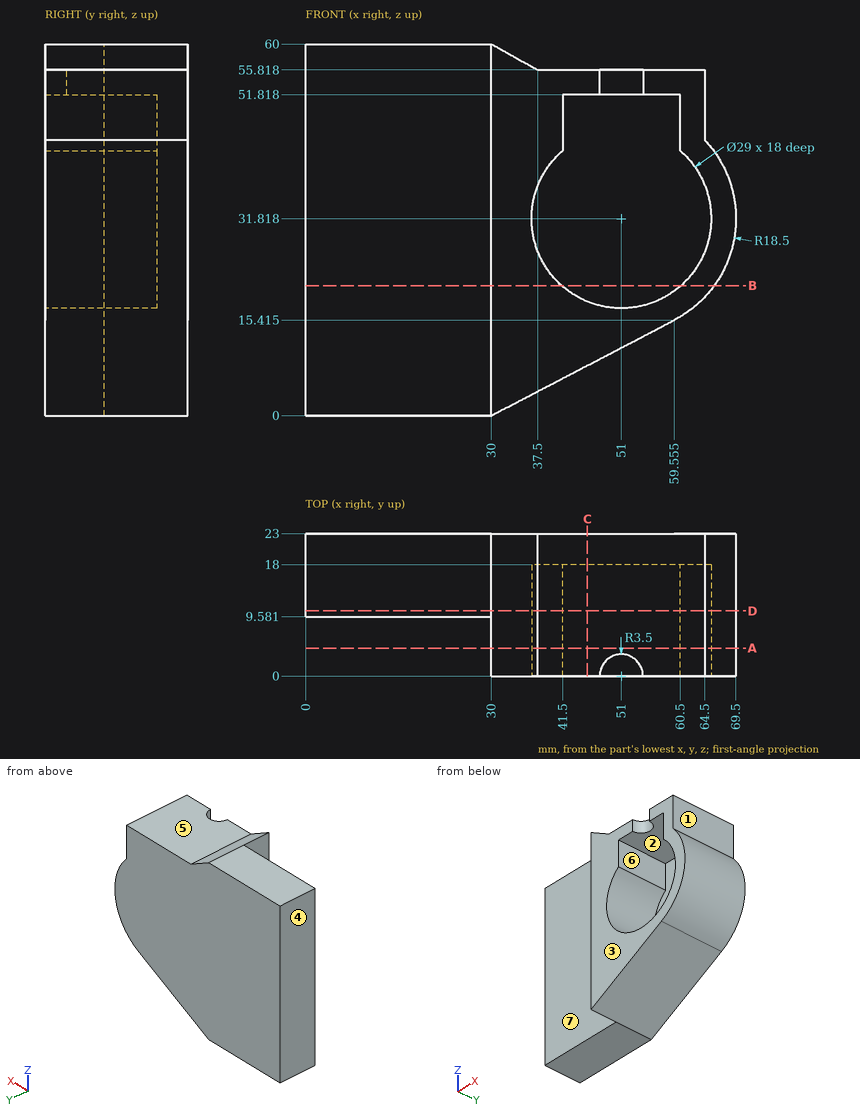
The drawing under review shows one solid part. Ordinate dimensions are in mm from its lowest x, y, z. A direction names the side the tool comes from. Give positions to 0.01 mm unless a question says otherwise; leave off trailing zeros. Write each loop counter-clockwise with the first axis right and the second up, starting at its lowest first coordinate (ties: lowest second). Pieces come first, ordered by that corner, then holes. Notation, with made-up numbers: (36.25, 33.5) - (53.25, 33.5) arc R11 ccw to (53.25, 48.5) - close; hole circle Ø9 at (65.25, 57). An arc over 180 degrees is marked (long way). Answer in a Markdown table with one row per item. Add a question column.
1. Tool access review of the marked faces 5, 6 and 7: name each direction out of +Z, -Z, +X, -X, +Y, -Y from which nothing blocks a thin tool from reaching the whole face with its end or side.
2. We need section C-C on x = 45.5. Write out the cut boundary in (y, z) (1 decimal).
3. Draft analysis for pull direction X (two halves, no side actions). For the marked faces 1, 2, 3 and 4, state which applies: +X half, -X half, draft (parallel to the pull), parting line (faces both ways), or undercut.
4. We need section B-B on z = 21. Write out the cut boundary in (x, y) (1 decimal).
5. We need section A-A on y = 4.5. Write out the cut boundary in (x, z) (1 decimal), then the cut area to 3 significant figures.
6. We need section D-D on y = 10.5. Write out the cut boundary in (x, z) (1 decimal), then the cut area to 3 significant figures.
7. Insertion check: P1, Ø3, axis at x = 33, z = 32.5, coming from the -Y side; P2, Ø3.5, axis at y = 14.5, z = 50.5, coming from the +X side; P3, Ø2.5, axis at y = 5.5, z = 48, coming from the -X side; P4, Ø11.5, axis at x = 48, y = 10.5, coming from the +Z side. Each pin has a flat end and moves straight along its axis. Give the tip position at first contact, or say it passes through.
8. Wall thickness on line 1 along X through (y, z) = (5.75, 48); line 2 along X through (y, z) = (21.25, 54); line 3 along Z through (x, y) = (38, 2) (1 decimal): over which ranges is each line inside the solid? List them lowest first. Write a range as [from, to].
Ans:
| question | item | result |
|---|---|---|
| 1 | face 5 | +Z, +X, +Y, -Y |
| 1 | face 6 | -Y |
| 1 | face 7 | +Z, -Z, -X, -Y |
| 2 | outline | (0, 8.1) - (23, 8.1) - (23, 55.8) - (0, 55.8) - (0, 51.8) - (18, 51.8) - (18, 18.4) - (0, 18.4) - close |
| 3 | face 1 | +X half |
| 3 | face 2 | undercut |
| 3 | face 3 | draft |
| 3 | face 4 | -X half |
| 4 | outline | (0, 9.6) - (30, 9.6) - (30, 0) - (41.3, 0) - (41.3, 18) - (60.7, 18) - (60.7, 0) - (66, 0) - (66, 23) - (0, 23) - close |
| 5 | outline | (30, 0) - (59.6, 15.4) arc R18.5 ccw to (64.5, 44.5) - (64.5, 55.8) - (37.5, 55.8) - (30, 60) - close; hole (41.5, 42.8) arc R14.5 ccw (long way) to (60.5, 42.8) - (60.5, 51.8) - (41.5, 51.8) - close |
| 5 | area | 930 mm^2 |
| 6 | outline | (0, 0) - (30, 0) - (59.6, 15.4) arc R18.5 ccw to (64.5, 44.5) - (64.5, 55.8) - (37.5, 55.8) - (30, 60) - (0, 60) - close; hole (41.5, 42.8) arc R14.5 ccw (long way) to (60.5, 42.8) - (60.5, 51.8) - (41.5, 51.8) - close |
| 6 | area | 2,730 mm^2 |
| 7 | P1 | stops at y = 0 |
| 7 | P2 | stops at x = 64.5 |
| 7 | P3 | stops at x = 30 |
| 7 | P4 | stops at z = 55.82 |
| 8 | line 1 | x = [30, 41.5], [60.5, 64.5] |
| 8 | line 2 | x = [0, 64.5] |
| 8 | line 3 | z = [4.2, 25.4], [38.2, 55.8] |
